Could you check a few things on this model? Use its own coordinates, in mm. A direction names the side the tool comes from. Give positions to 0.01 mm unless a question says otherwise; leave off trailing zeros. Write each loop counter-clockwise with the first axis right and the second up, starting at its lowest first coordinate (ties: lowest second). Pieces come first, ordered by that corner, then holes. Notation, with made-up numbers: (-14, -14.75) -> (1, -14.75) arc R23 ccw to (1, -1.75) -> close; hole circle Ø7 at (35, 59.25). An arc over 180 degrees is marked (long way). One line per question, with ' | ' between items.
from build123d import *

# Parameters (mm, degrees)
SKETCH1_W           = 52
SKETCH1_H           = 32
BOSS_EXTRUDE1_DEPTH = 10
SKETCH7_W           = 4.5
SKETCH7_H           = 40
CUT_EXTRUDE3_DEPTH  = 33
SKETCH70_W          = 5.5
SKETCH70_H          = 44.25
BOSS_EXTRUDE4_DEPTH = 20
SKETCH20_W          = 5.5
SKETCH20_H          = 33.25
CUT_EXTRUDE9_DEPTH  = 21
FILLET1_R           = 6
FILLET2_R           = 6
SKETCH49_W          = 4.5
SKETCH49_H          = 32
BOSS_EXTRUDE3_DEPTH = 12.5
SKETCH50_W          = 4.5
SKETCH50_H          = 24.5
CUT_EXTRUDE19_DEPTH = 3
SKETCH35_W          = 9
SKETCH35_H          = 25.742086546
CUT_EXTRUDE15_DEPTH = 6.5
SKETCH67_W          = 5
SKETCH67_H          = 25.742086546
CUT_EXTRUDE22_DEPTH = 3
SKETCH68_W          = 5
SKETCH68_H          = 25.742086546
CUT_EXTRUDE23_DEPTH = 3
SKETCH63_W          = 6
SKETCH63_H          = 22
CUT_EXTRUDE24_DEPTH = 11
SKETCH76_W          = 10.5
SKETCH76_H          = 22
CUT_EXTRUDE25_DEPTH = 7


with BuildPart() as part:
    # Sketch1 → Boss-Extrude1 (new body)
    with BuildSketch(Plane(origin=(0, 0, 0), x_dir=(0, 0, -1), z_dir=(1, 0, 0))):
        Rectangle(SKETCH1_W, SKETCH1_H)
    extrude(amount=BOSS_EXTRUDE1_DEPTH)

    # Sketch7 → Cut-Extrude3 (cut, through all)
    with BuildSketch(Plane(origin=(0, 16, 0), x_dir=(1, 0, 0), z_dir=(0, 1, 0))):
        with Locations((2.25, 6)):
            Rectangle(SKETCH7_W, SKETCH7_H)
    extrude(amount=-CUT_EXTRUDE3_DEPTH, mode=Mode.SUBTRACT)

    # Sketch70 → Boss-Extrude4 (add)
    with BuildSketch(Plane(origin=(0, -16, 0), x_dir=(-1, 0, 0), z_dir=(0, -1, 0))):
        with Locations((-7.25, 3.875)):
            Rectangle(SKETCH70_W, SKETCH70_H)
    extrude(amount=BOSS_EXTRUDE4_DEPTH)

    # Sketch20 → Cut-Extrude9 (cut, through all)
    with BuildSketch(Plane(origin=(0, -16, 0), x_dir=(-1, 0, 0), z_dir=(0, -1, 0))):
        with Locations((-7.25, 3.875)):
            Rectangle(SKETCH20_W, SKETCH20_H)
    extrude(amount=CUT_EXTRUDE9_DEPTH, mode=Mode.SUBTRACT)

    # Fillet1
    fillet1_edges = [part.edges().sort_by_distance(p)[0] for p in [
        (7.25, -16, -20.5),
    ]]
    fillet(fillet1_edges, radius=FILLET1_R)

    # Fillet2
    fillet2_edges = [part.edges().sort_by_distance(p)[0] for p in [
        (7.25, -16, 12.75),
    ]]
    fillet(fillet2_edges, radius=FILLET2_R)

    # Sketch49 → Boss-Extrude3 (add)
    with BuildSketch(Plane(origin=(0, 0, 14), x_dir=(-1, 0, 0), z_dir=(0, 0, -1))):
        with Locations((-2.25, 0)):
            Rectangle(SKETCH49_W, SKETCH49_H)
    extrude(amount=BOSS_EXTRUDE3_DEPTH)

    # Sketch50 → Cut-Extrude19 (cut)
    with BuildSketch(Plane.XZ.offset(16)):
        with Locations((2.25, 13.75)):
            Rectangle(SKETCH50_W, SKETCH50_H)
    extrude(amount=-CUT_EXTRUDE19_DEPTH, mode=Mode.SUBTRACT)

    # Sketch35 → Cut-Extrude15 (cut, through all)
    with BuildSketch(Plane.ZY.offset(-4.5)):
        with Locations((-9.381446742, 0.030527838)):
            Rectangle(SKETCH35_W, SKETCH35_H)
    extrude(amount=-CUT_EXTRUDE15_DEPTH, mode=Mode.SUBTRACT)

    # Sketch67 → Cut-Extrude22 (cut)
    with BuildSketch(Plane.ZY.offset(-4.5)):
        with Locations((-18.381446742, 0.030527838)):
            Rectangle(SKETCH67_W, SKETCH67_H)
    extrude(amount=-CUT_EXTRUDE22_DEPTH, mode=Mode.SUBTRACT)

    # Sketch68 → Cut-Extrude23 (cut)
    with BuildSketch(Plane.ZY.offset(-4.5)):
        with Locations((-0.381446742, 0.030527838)):
            Rectangle(SKETCH68_W, SKETCH68_H)
    extrude(amount=-CUT_EXTRUDE23_DEPTH, mode=Mode.SUBTRACT)

    # Sketch63 → Cut-Extrude24 (cut, through all)
    with BuildSketch(Plane.ZY):
        with Locations((20, 1)):
            Rectangle(SKETCH63_W, SKETCH63_H)
    extrude(amount=-CUT_EXTRUDE24_DEPTH, mode=Mode.SUBTRACT)

    # Sketch76 → Cut-Extrude25 (cut)
    with BuildSketch(Plane.ZY):
        with Locations((9.75, 1)):
            Rectangle(SKETCH76_W, SKETCH76_H)
    extrude(amount=-CUT_EXTRUDE25_DEPTH, mode=Mode.SUBTRACT)


with BuildPart() as body_2:
    # Mirror1: mirrored copy
    add(part.part.mirror(Plane(origin=(10, 16, 26), x_dir=(1, 0, 0), z_dir=(0, 0, -1))))


solid = body_2.part
Q1. Imagine slicing it at D-D on x = 3.5. Please give me the cut outline in (y, z), and give its area (4 significant figures).
Answer below:
outline: (-13, 26) -> (16, 26) -> (16, 50.5) -> (-13, 50.5) -> close; hole (-10, 29) -> (12, 29) -> (12, 35) -> (-10, 35) -> close; hole (-10, 37) -> (12, 37) -> (12, 47.5) -> (-10, 47.5) -> close | area: 347.5 mm^2
Q2. Will these pins go through, and if not, where does the flat tip stop? pin 1 (1.3 mm diameter, centred on x = 1.5, z = 43.5, fed in from -Y); pin 2 (1.6 mm diameter, centred on x = 7, z = 31, fed in from -Y); pin 3 (2 mm diameter, centred on y = -6.5, z = 45, fed in from -X).
Answer below:
pin 1: stops at y = -13 | pin 2: stops at y = -16 | pin 3: stops at x = 7
Q3. If I drill on line 1 along Z through (x, y) = (8, -3.5); line 2 along Z through (x, y) = (2, 2.5); line 3 along Y through (x, z) = (3.5, 38), over which ranges is the centre line in solid material (lowest first)?
Answer below:
line 1: z = 26 to 29, 35 to 56.88, 65.88 to 78 | line 2: z = 26 to 29, 35 to 37, 47.5 to 50.5 | line 3: y = -13 to -10, 12 to 16
Q4. Imagine slicing it at B-B on y = 6. Please give me the cut outline in (x, z), and give its area (3 significant figures).
Answer below:
outline: (0, 26) -> (10, 26) -> (10, 29) -> (0, 29) -> close; (0, 35) -> (10, 35) -> (10, 56.88) -> (4.5, 56.88) -> (4.5, 54.88) -> (7.5, 54.88) -> (7.5, 49.88) -> (4.5, 49.88) -> (4.5, 50.5) -> (0, 50.5) -> (0, 47.5) -> (7, 47.5) -> (7, 37) -> (0, 37) -> close; (4.5, 65.88) -> (10, 65.88) -> (10, 78) -> (4.5, 78) -> (4.5, 72.88) -> (7.5, 72.88) -> (7.5, 67.88) -> (4.5, 67.88) -> close | area: 183 mm^2
Q5. Imagine slicing it at C-C on y = -24. Please give me the cut outline in (x, z).
Answer below:
outline: (4.5, 33.75) -> (10, 33.75) -> (10, 39.25) -> (4.5, 39.25) -> close; (4.5, 72.5) -> (10, 72.5) -> (10, 78) -> (4.5, 78) -> close
Q6. Imagine slicing it at A-A on z = 63.5. Please give me the cut outline in (x, y), and give its area (3 significant figures).
Answer below:
outline: (4.5, -16) -> (10, -16) -> (10, -12.84) -> (4.5, -12.84) -> close; (4.5, 12.9) -> (10, 12.9) -> (10, 16) -> (4.5, 16) -> close | area: 34.4 mm^2
Q7. If we mould it in two halves opening along Z, with no side actions, what happens to faces 1 (the flat face through (5, 0, 26)), 2 (the flat face through (7, -36, 37)), 3 (the flat face through (6, -12.841, 52))? For each: +Z half, -Z half, draft (parallel to the pull), parting line (faces both ways), or undercut.
Answer below:
face 1: -Z half | face 2: draft | face 3: undercut
Q8. On a 3-axis mill with a long thin cutter (end or side, diameter ignored), from which of +Z, -Z, +X, -X, +Y, -Y can I reach the whole of each face in a straight line? I mean faces 4 (the flat face through (7, 0, 56.881)), 5 (the flat face through (7, -29, 39.25)), 6 (the flat face through (3, 1, 37)). Say none if no direction works.
Answer below:
face 4: +X, -X | face 5: +X, -X, -Y | face 6: -X
